Design review of the part built by this model. Coordinates are the model's own, in mm. A direction names the side the tool comes from. Coordinates: 2 decimals unless noted, no trailing zeros. Loops run counter-clockwise (first coordinate to the right, second up) from the corner with the lowest first, then second, coordinate; pieces in that order, holes last. Notation, with made-up numbers: (-32.75, 23) -> (7.25, 23) arc R14 ccw to (7.25, 27) -> close; hole circle Ø5 at (75.5, 87.25). An arc over 180 degrees is marked (long way). Answer as a JSON object with one key per item and string values.
```python
from build123d import *

# Parameters (mm, degrees)
F8_W      = 60.2088514067
F8_H      = 41.021
F9_DEPTH  = 1.524
F6_R      = 3.3655
F6_R_2    = 2.0955
F7_R      = 3.3655
F7_R_2    = 2.0955
F10_DEPTH = 4.064
F11_DEPTH = 25.4


with BuildPart() as f9:
    # F8 (on Top) → F9 (new body)
    with BuildSketch(Plane.XY):
        Rectangle(F8_W, F8_H)
    extrude(amount=F9_DEPTH)

    # F6 (on face) + F7 (on face) → F10 (join)
    with BuildSketch(Plane.XY):
        with Locations((-23.9141, -15.367)):
            Circle(F6_R)
        with Locations((-23.9141, -15.367)):
            Circle(F6_R_2, mode=Mode.SUBTRACT)
    with BuildSketch(Plane.XY):
        with Locations((23.9141, 15.367)):
            Circle(F7_R)
        with Locations((23.9141, 15.367)):
            Circle(F7_R_2, mode=Mode.SUBTRACT)
    extrude(amount=F10_DEPTH)

    # F11 (cut): faces of the model
    f11_faces = [f9.faces().sort_by_distance(p)[0] for p in [
        (-23.9141, -15.367, 1.524),
        (23.9141, 15.367, 1.524),
    ]]
    extrude(f11_faces, amount=-F11_DEPTH, mode=Mode.SUBTRACT)


solid = f9.part
```
1) Add section A-A, the plane y = -16.5. Give the boundary of the cut face in (x, z).
Completed:
{"outline": "(-30.1, 0) -> (-25.68, 0) -> (-25.68, 4.06) -> (-27.08, 4.06) -> (-27.08, 1.52) -> (-30.1, 1.52) -> close; (-22.15, 0) -> (30.1, 0) -> (30.1, 1.52) -> (-20.75, 1.52) -> (-20.75, 4.06) -> (-22.15, 4.06) -> close"}
2) Wall thickness on probe 1 along X at (y, z) = (15.5, 2.25); probe 2 along Z at (x, y) = (21, -13); probe 3 along Y at (x, z) = (-22, 1.4): over which ranges is each line inside the solid? List them lowest first.
Completed:
{"probe 1": "20.55 to 21.82, 26.01 to 27.28", "probe 2": "0 to 1.52", "probe 3": "-20.51 to -16.22, -14.51 to 20.51"}
3) Add section B-B, the plane z = 2.45. Give the boundary of the cut face in (x, y), and give its area (3 significant figures).
Completed:
{"outline": "circle Ø6.73 at (-23.91, -15.37); circle Ø6.73 at (23.91, 15.37); hole circle Ø4.19 at (-23.91, -15.37); hole circle Ø4.19 at (23.91, 15.37)", "area": "43.6 mm²"}
4) For faces 4 (the flat face through (-22, -14, 4.064)), 5 (the cylindrical face through (27.023, 14.078, 2.776)), list the 3-axis set-ups (+Z, -Z, +X, -X, +Y, -Y) from which the entire face can be reached by the end or side of a thin tool; tool diameter is ignored.
Completed:
{"face 4": "+Z, +X, -X, +Y, -Y", "face 5": "+Z"}
5) Clearance check with flat-ended pins moving along their axes: pin 1 Ø6.5 at (x, y) = (23.91, 15.37) entering from -Z; pin 2 Ø3 at (x, y) = (-4, -6) entering from +Z; pin 3 Ø4 at (x, y) = (-23.91, -15.37) entering from +Z. State where each tip first meets the part, or that it passes through.
Completed:
{"pin 1": "z = 0", "pin 2": "z = 1.52", "pin 3": "through"}
6) Add section D-D, the plane x = 0. Give the boundary of the cut face in (y, z), and give its area (3 significant figures).
Completed:
{"outline": "(-20.51, 0) -> (20.51, 0) -> (20.51, 1.52) -> (-20.51, 1.52) -> close", "area": "62.5 mm²"}
7) The part is to be moulded in two halves that separate along Y. For faces 1 (the cylindrical face through (-24.37, -13.32, 2.06)), 2 (the cylindrical face through (-20.805, -16.656, 2.776)), 3 (the flat face through (0, 0, 1.524)), say which applies: pulls with the +Y half, pulls with the -Y half, needs draft (parallel to the pull), parting line crosses it, or undercut.
Completed:
{"face 1": "undercut", "face 2": "parting line crosses it", "face 3": "needs draft"}
8) Add section C-C, the plane y = -3. Give the boundary of the cut face in (x, z), and give its area (3 significant figures).
Completed:
{"outline": "(-30.1, 0) -> (30.1, 0) -> (30.1, 1.52) -> (-30.1, 1.52) -> close", "area": "91.8 mm²"}
